Can you work these out from the drawing? Everything is in mm from the part's minimum corner. A direction names the side the tool comes from. Give positions to 0.01 mm unless a question says otherwise; leave off trailing zeros. Order: outer loops, then holes, each group sorted by start corner. A loop starts at its lowest first (then second) coordinate and runs counter-clockwise, first axis right, second up. Notation, with made-up numbers: (19.25, -28.5) - (38.25, -28.5) arc R19 ccw to (38.25, 7.5) - close; hole circle Ø1 at (42, -10.5). An arc over 180 degrees is marked (long way). Answer as a JSON object with one key per item and string values.
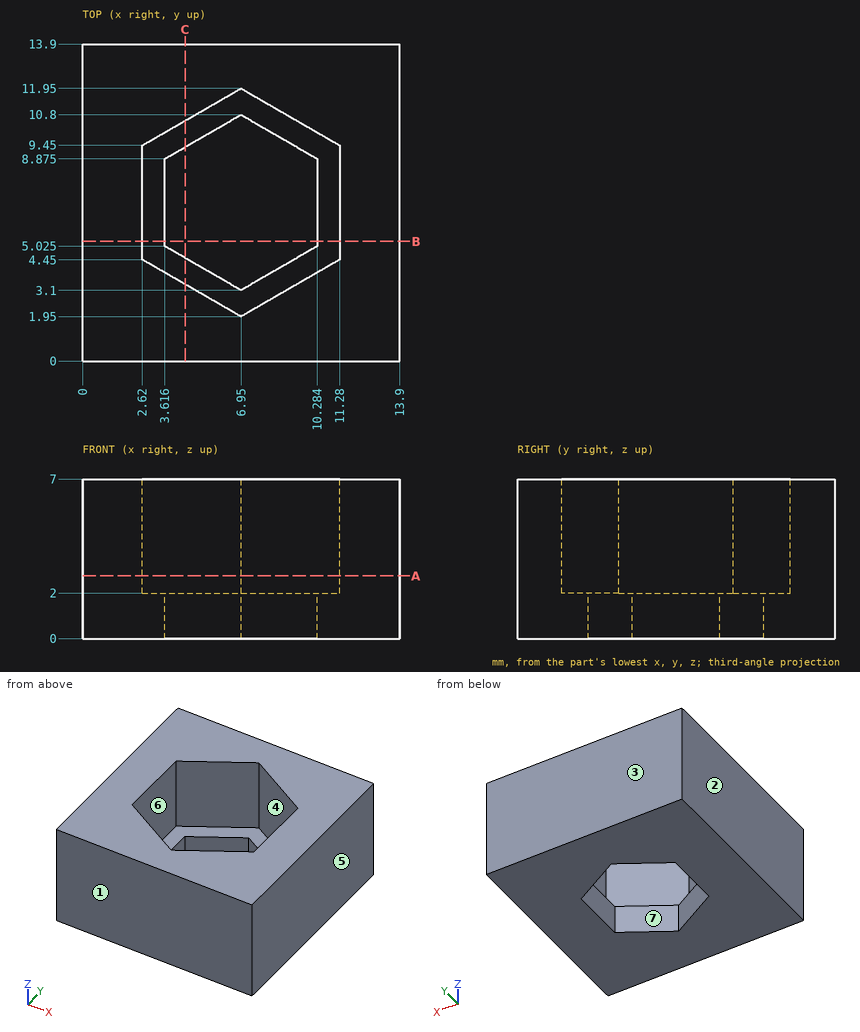
Q1. If we section it at C-C, the plane x = 4.5: Please give me the cut outline in (y, z).
Recorded:
{"outline": "(0, 0) - (4.51, 0) - (4.51, 2) - (3.36, 2) - (3.36, 7) - (0, 7) - close; (9.39, 0) - (13.9, 0) - (13.9, 7) - (10.54, 7) - (10.54, 2) - (9.39, 2) - close"}
Q2. I need wall thicknesses on L1, parallel to X at y = 4.5, z = 2.25; L2, parallel to Y at x = 7.25, z = 0.5; L3, parallel to Y at x = 6.75, z = 3 (1 decimal). Which ranges of each line are inside material? Lowest first, please.
Recorded:
{"L1": "x = 0 to 2.62, 11.28 to 13.9", "L2": "y = 0 to 3.27, 10.63 to 13.9", "L3": "y = 0 to 2.1, 11.8 to 13.9"}
Q3. If we section it at B-B, the plane y = 5.25: Please give me the cut outline in (x, z).
Recorded:
{"outline": "(0, 0) - (3.62, 0) - (3.62, 2) - (2.62, 2) - (2.62, 7) - (0, 7) - close; (10.28, 0) - (13.9, 0) - (13.9, 7) - (11.28, 7) - (11.28, 2) - (10.28, 2) - close"}
Q4. We'd pull the mould along Y, two halves only. Please class the marked faces 1, 2, 3 and 4: released by +Y, released by -Y, zero draft, split by the parting line, or undercut.
Recorded:
{"face 1": "released by -Y", "face 2": "zero draft", "face 3": "released by +Y", "face 4": "undercut"}
Q5. Which directions (+Z, -Z, +X, -X, +Y, -Y) give clear straight access to the entire face, cutting with the end or side of a thin tool? Please do the marked faces 5, 6 and 7.
Recorded:
{"face 5": "+Z, -Z, +X, +Y, -Y", "face 6": "+Z", "face 7": "+Z, -Z"}
Q6. If we section it at A-A, the plane z = 2.75: Please give me the cut outline in (x, y).
Recorded:
{"outline": "(0, 0) - (13.9, 0) - (13.9, 13.9) - (0, 13.9) - close; hole (2.62, 4.45) - (6.95, 1.95) - (11.28, 4.45) - (11.28, 9.45) - (6.95, 11.95) - (2.62, 9.45) - close"}
